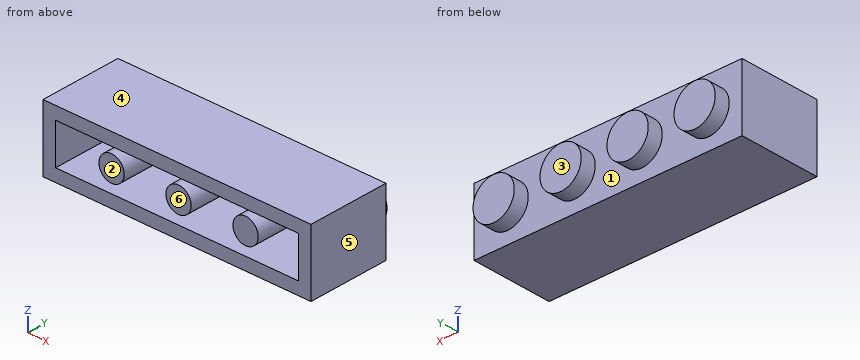
from build123d import *

# Parameters (mm, degrees)
SKETCH2_W           = 31.81
SKETCH2_H           = 7.81
BOSS_EXTRUDE1_DEPTH = 9.65
SKETCH3_R           = 2.45
BOSS_EXTRUDE2_DEPTH = 1.8
SHELL1_T            = -1.5
SKETCH4_R           = 1.5
BOSS_EXTRUDE3_DEPTH = 7.95


with BuildPart() as part:
    # Sketch2 → Boss-Extrude1 (new body)
    with BuildSketch(Plane(origin=(0, 0, 0), x_dir=(1, 0, 0), z_dir=(0, 1, 0))):
        Rectangle(SKETCH2_W, SKETCH2_H)
    extrude(amount=-BOSS_EXTRUDE1_DEPTH)

    # Sketch3 → Boss-Extrude2 (add)
    with BuildSketch(Plane(origin=(0, 0, 0), x_dir=(1, 0, 0), z_dir=(0, 1, 0))):
        with Locations(Location((-11.92875, 0, 0), (0, 0, 270))):
            Circle(SKETCH3_R)
        with Locations(Location((-3.97625, 0, 0), (0, 0, 270))):
            Circle(SKETCH3_R)
        with Locations(Location((3.97625, 0, 0), (0, 0, 270))):
            Circle(SKETCH3_R)
        with Locations(Location((11.92875, 0, 0), (0, 0, 270))):
            Circle(SKETCH3_R)
    extrude(amount=BOSS_EXTRUDE2_DEPTH)

    # Shell1
    shell1_openings = [part.faces().sort_by_distance(p)[0] for p in [
        (0, -9.65, 0),
    ]]
    offset(amount=SHELL1_T, openings=shell1_openings, kind=Kind.INTERSECTION)

    # Sketch4 → Boss-Extrude3 (add)
    with BuildSketch(Plane.XZ.offset(1.5)):
        with Locations(Location((-7.9525, 0, 0), (0, 0, 90))):
            Circle(SKETCH4_R)
        with Locations(Location((0, 0, 0), (0, 0, 90))):
            Circle(SKETCH4_R)
        with Locations(Location((7.9525, 0, 0), (0, 0, 90))):
            Circle(SKETCH4_R)
    extrude(amount=BOSS_EXTRUDE3_DEPTH)


solid = part.part
The listing builds one solid part. Answer for the finished solid, in the listing's coordinates (mm). Face numbers are marked on the shaded views. A direction names the side the tool comes from. Round coordinates to 2 decimals unless told otherwise and drop trailing zeros. Write each loop counter-clockwise with the first axis right and the second up, starting at its lowest first coordinate (ties: lowest second). Pieces come first, ordered by that corner, then holes. Notation, with made-up numbers: (51, 4.5) - (78, 4.5) arc R23 ccw to (78, 12.5) - close; hole circle Ø3 at (49.25, 80.25). An arc over 180 degrees is marked (long way). Use a Markdown table: item, result. Add a question column.
1. The part is cut by section A-A (y = -5). Write down the section's boundary in (x, z) (1 decimal).
2. Consider line 1 (Z direction, x = -8, y = -2.25) (3 decimals); line 2 (X direction, y = -0.15, z = 0) (3 decimals); line 3 (X direction, y = -8, z = 1.75) (3 decimals). Determine where each line is inside the solid, lowest interval first.
3. A tool of negligible diameter and unlimited length cuts with its end or side. For the marked faces 1, 2 and 3, from which of +Z, -Z, +X, -X, +Y, -Y can it reach the whole face along a straight path? Write none if from no direction.
4. For a pull along Z with two mould halves and no side action, classify the marked faces 4, 5 and 6 as +Z half, -Z half, draft (parallel to the pull), parting line (faces both ways), or undercut.
5. Flat-ended cylindrical pins translate along their axes: P1, Ø2, axis at x = -5.5, y = 0.5, coming from the -Z side (3 decimals); P2, Ø0.9, axis at x = 8.5, z = -0.5, coming from the -Y side; P3, Ø0.9, axis at x = 11.5, z = -0.5, coming from the -Y side; P4, Ø1, axis at x = -4, z = 0, coming from the -Y side. Find the tip coordinate at first contact, or state that the pin passes through.
6. The part is cut by section B-B (x = 0). Write down the section's boundary in (y, z) (3 decimals), and give its area (3 significant figures).
7. The part is cut by section C-C (z = -3.25). Write down the section's boundary in (x, y) (3 decimals).
Reported:
| question | item | result |
|---|---|---|
| 1 | outline | (-15.9, -3.9) - (15.9, -3.9) - (15.9, 3.9) - (-15.9, 3.9) - close; circle Ø3 at (-8, 0); circle Ø3 at (0, 0); circle Ø3 at (8, 0); hole (-14.4, -2.4) - (14.4, -2.4) - (14.4, 2.4) - (-14.4, 2.4) - close |
| 2 | line 1 | -3.905 to -2.405, -1.499 to 1.499, 2.405 to 3.905 |
| 2 | line 2 | -15.905 to -12.879, -10.979 to -4.926, -3.026 to 3.026, 4.926 to 10.979, 12.879 to 15.905 |
| 2 | line 3 | -15.905 to -14.405, 14.405 to 15.905 |
| 3 | face 1 | +Y |
| 3 | face 2 | -Y |
| 3 | face 3 | +Z, -Z, +X, -X, +Y |
| 4 | face 4 | +Z half |
| 4 | face 5 | draft |
| 4 | face 6 | undercut |
| 5 | P1 | z = -3.905 |
| 5 | P2 | y = -9.45 |
| 5 | P3 | y = -1.5 |
| 5 | P4 | y = 0.3 |
| 6 | outline | (-9.65, -3.905) - (0, -3.905) - (0, 3.905) - (-9.65, 3.905) - (-9.65, 2.405) - (-1.5, 2.405) - (-1.5, 1.5) - (-9.45, 1.5) - (-9.45, -1.5) - (-1.5, -1.5) - (-1.5, -2.405) - (-9.65, -2.405) - close |
| 6 | area | 60.0 mm^2 |
| 7 | outline | (-15.905, -9.65) - (15.905, -9.65) - (15.905, 0) - (-15.905, 0) - close |
